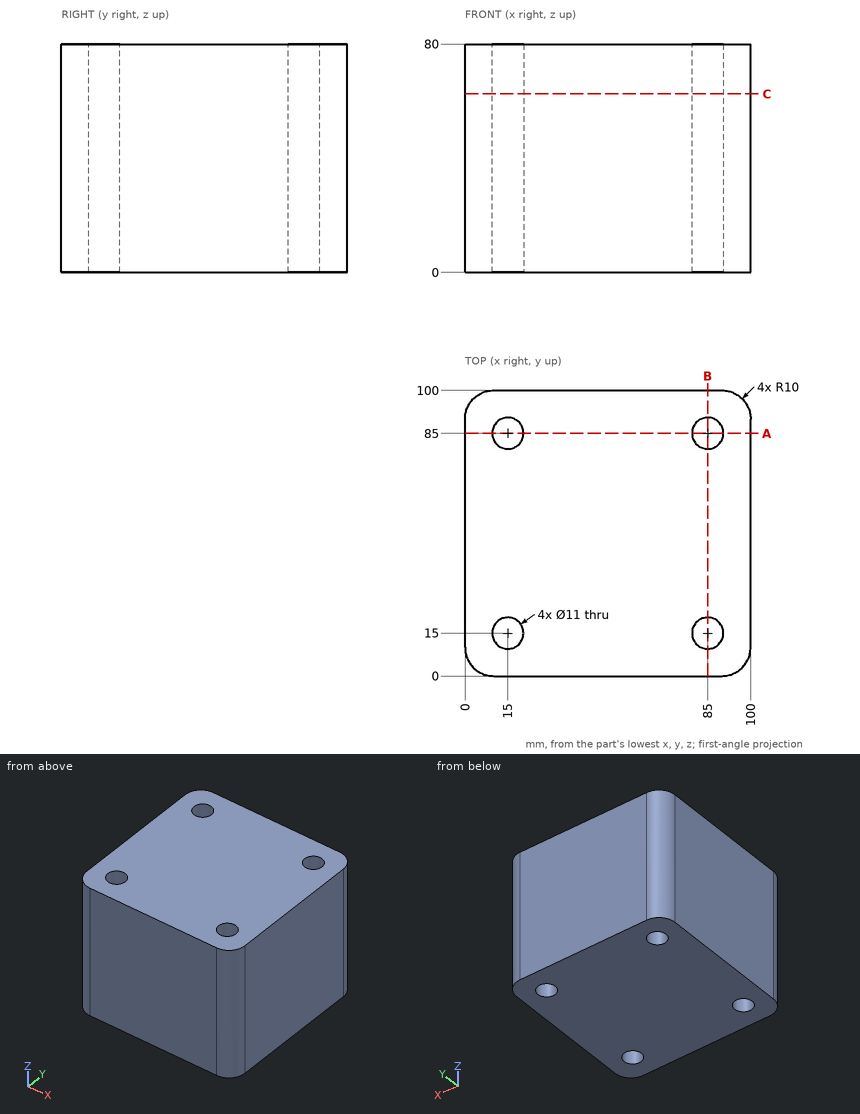
Part print with two shaded views. Sizes in mm from the minimum x, y, z corner. Coordinates: 2 decimals unless noted, no trailing zeros. Loops run counter-clockwise (first coordinate to the right, second up) from the corner with the lowest first, then second, coordinate; pieces in that order, holes last. Notation, with made-up numbers: (40.25, 18) - (88.25, 18) arc R11 cw to (88.25, 38) - close; hole circle Ø9 at (41, 29). An arc over 180 degrees is marked (long way). Write each question's results on one line, items separated by ' | '. Start each with the question number.
Q1. Slice it at A-A on y = 85. Give the cut face in (x, z).
Q2. Slice it at C-C on z = 62.5. Give the cut face in (x, y).
Q3. Probe line 1 along Y through (x, z) = (85, 44.5); line 2 along X through (y, z) = (85.5, 60); line 3 along X through (y, z) = (18.5, 75). List the from-to ranges inside material, lowest first.
Q4. Drop flat-ended pins along their axis: pin 1 Ø10 at (x, y) = (85, 15) entering from +Z; pin 2 Ø3 at (x, y) = (89, 83.5) entering from -Z. Give the stop position or say it passes through.
Answer:
1) outline: (0, 0) - (9.5, 0) - (9.5, 80) - (0, 80) - close; (20.5, 0) - (79.5, 0) - (79.5, 80) - (20.5, 80) - close; (90.5, 0) - (100, 0) - (100, 80) - (90.5, 80) - close
2) outline: (0, 10) arc R10 ccw to (10, 0) - (90, 0) arc R10 ccw to (100, 10) - (100, 90) arc R10 ccw to (90, 100) - (10, 100) arc R10 ccw to (0, 90) - close; hole circle Ø11 at (15, 15); hole circle Ø11 at (15, 85); hole circle Ø11 at (85, 15); hole circle Ø11 at (85, 85)
3) line 1: y = 0 to 9.5, 20.5 to 79.5, 90.5 to 100 | line 2: x = 0 to 9.52, 20.48 to 79.52, 90.48 to 100 | line 3: x = 0 to 10.76, 19.24 to 80.76, 89.24 to 100
4) pin 1: passes through | pin 2: stops at z = 0
